```python
from build123d import *

# Parameters (mm, degrees)
F0_W     = 142.24
F0_H     = 38.1
F1_DEPTH = 73
F3_DEPTH = 142.24
F4_DEPTH = 12.7


with BuildPart() as f1:
    # F0 (on Top) → F1 (new body)
    with BuildSketch(Plane.XY):
        with Locations((2.9369369149, 17.2356535431)):
            Rectangle(F0_W, F0_H)
    extrude(amount=F1_DEPTH)

    # F2 (on face) → F3 (cut)
    with BuildSketch(Plane(origin=(-68.1830630851, 0, 0), x_dir=(0, -1, 0), z_dir=(-1, 0, 0))):
        with BuildLine():
            Line((-36.2856535431, 63.1459391326), (-36.2856535431, 50.6160780787))
            ThreePointArc((-36.2856535431, 50.6160780787), (-28.8997261841, 56.8810086057), (-36.2856535431, 63.1459391326))
        make_face()
    extrude(amount=-F3_DEPTH, mode=Mode.SUBTRACT)

    # F4 (cut): a face of the model
    f4_faces = [f1.faces().sort_by_distance(p)[0] for p in [
        (2.9369369149, -1.8143464569, 36.5),
    ]]
    extrude(f4_faces, amount=-F4_DEPTH, mode=Mode.SUBTRACT)


solid = f1.part
```
The listing builds one solid part. Answer for the finished solid, in the listing's coordinates (mm). Round coordinates to 2 decimals unless told otherwise and drop trailing zeros. Loops run counter-clockwise (first coordinate to the right, second up) from the corner with the lowest first, then second, coordinate; pieces in that order, holes last. Notation, with made-up numbers: (-28.5, -9) - (-20.5, -9) arc R24 cw to (-20.5, 25) - close; hole circle Ø3 at (11.25, 48.5). An arc over 180 degrees is marked (long way). Use one line per item in the form item = value. Start each with the question number.
1. Given pin 1 Ø3 at (y, z) = (33.5, 60.5) entering from +X, flat-ended and moving along its own axis, determine where the tip first touches the part or whether it passes through.
2. For a pull along Z with two mould halves and no side action, classify faces 1 (the face through (2, 24, 73)), 2 (the face through (2, 36.286, 25)), 3 (the face through (2, 24, 0)), 4 (the face through (1.94, 28.9, 56.73)) as pulls with the +Z half, pulls with the -Z half, needs draft (parallel to the pull), parting line crosses it, or undercut.
3. Consider line 1 (Z direction, x = -7.5, y = 33.5); line 2 (Z direction, x = 58.5, y = 31); line 3 (Y direction, x = 35.5, z = 59.5). Determine where each line is inside the solid, lowest interval first. Write a range as [from, to].
4. The part is cut by section A-A on x = 43.5. Determine the outline of the cut face in (y, z).
Geometry check:
q1.pin_1 = through
q2.face_1 = pulls with the +Z half
q2.face_2 = needs draft
q2.face_3 = pulls with the -Z half
q2.face_4 = undercut
q3.line_1 = [0, 50.78], [62.99, 73]
q3.line_2 = [0, 52.16], [61.6, 73]
q3.line_3 = [10.89, 29.46]
q4.outline = (10.89, 0) - (36.29, 0) - (36.29, 50.62) arc R6.35 cw (long way) to (36.29, 63.15) - (36.29, 73) - (10.89, 73) - close
